Geometry: see drawing. Coordinates: mm, zero at the bounding-box minimum. A direction names the side the tool comes from. Coordinates: 2 decimals unless noted, no trailing zeros. Write each loop counter-clockwise with the first axis right and the second up, starting at its lowest first coordinate (ties: lowest second). Pieces come first, ordered by that corner, then holes. Notation, with made-up numbers: M 30.25,-37 L 34.25,-37 A13 cw 34.25,-27 Z; hole C 61,-35 d9. An arc over 180 degrees is marked long. Write item = value, one per line. Start each with the question number.
1. Section query C-C (y = 134.5). Output: boundary loops of the cut face in (x, z), then the cut area to 3 significant figures.
2. Section query A-A (x = 5). Output: boundary loops of the cut face in (y, z).
3. Access query for the marked faces 1 and 2. Directions: +Z, -Z, +X, -X, +Y, -Y. A direction counts if a zero-diameter tool reaches every point of the face in a straight line with its end or side. Return the directions, or none.
4. Line query: line 1 along Y through (x, z) = (73, 15); line 2 along X through (y, z) = (193, 7.5); line 3 along Z through (x, y) = (23.5, 202.5). Output: solid intervals per line, ascending.
5. Pull-direction query (X, two-part tool) for the marked faces 3, 4, 5 and 6; classes: pulls with the +X half, pulls with the -X half, needs draft (parallel to the pull), parting line crosses it, or undercut.
6. Section query B-B (z = 5). Output: boundary loops of the cut face in (x, y).
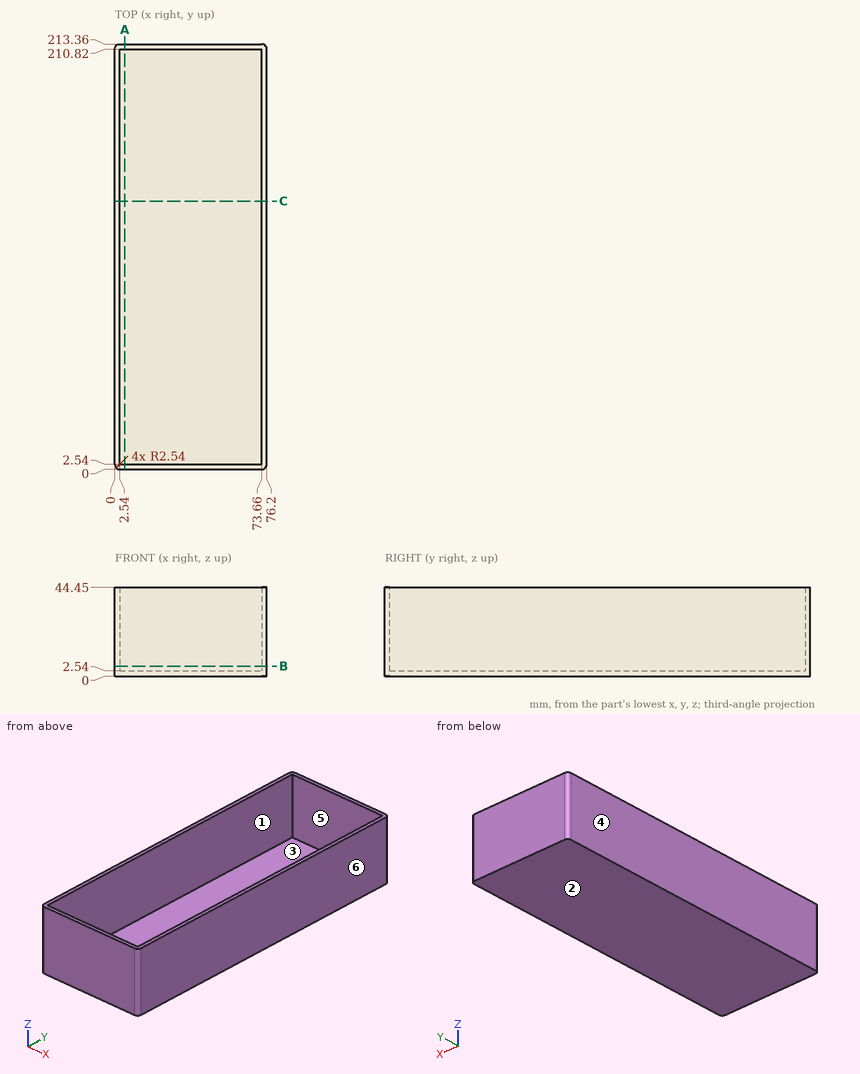
Results are:
q1.outline = M 0,0 L 76.2,0 L 76.2,44.45 L 73.66,44.45 L 73.66,2.54 L 2.54,2.54 L 2.54,44.45 L 0,44.45 Z
q1.area = 406 mm^2
q2.outline = M 0,0 L 213.36,0 L 213.36,44.45 L 210.82,44.45 L 210.82,2.54 L 2.54,2.54 L 2.54,44.45 L 0,44.45 Z
q3.face_1 = +Z
q3.face_2 = -Z, +X, -X, +Y, -Y
q4.line_1 = 0 to 2.54, 210.82 to 213.36
q4.line_2 = 0 to 2.54, 73.66 to 76.2
q4.line_3 = 0 to 2.54
q5.face_3 = undercut
q5.face_4 = pulls with the -X half
q5.face_5 = undercut
q5.face_6 = pulls with the +X half
q6.outline = M 0,2.54 A2.54 ccw 2.54,0 L 73.66,0 A2.54 ccw 76.2,2.54 L 76.2,210.82 A2.54 ccw 73.66,213.36 L 2.54,213.36 A2.54 ccw 0,210.82 Z; hole M 2.54,2.54 L 73.66,2.54 L 73.66,210.82 L 2.54,210.82 Z
